Here's how the part is built. I have some questions about the finished solid (model axes, mm). A direction names the side the tool comes from. Coordinates: 2 decimals unless noted, no trailing zeros. Loops run counter-clockwise (first coordinate to the right, second up) from the corner with the lowest first, then second, coordinate; pieces in that order, holes last. Notation, with made-up numbers: (59.5, 23.25) -> (68.5, 23.25) arc R20 ccw to (68.5, 62.25) -> close; hole circle Ø4 at (27.25, 40). An arc over 180 degrees is marked (long way). Answer as a JSON object with one key per item and string values. Group by question number.
Q1. I want a section at A-A on y = -34.75. Write out the boundary of the cut face in (x, z).
Q2. I want a section at D-D on y = -46.75. Write out the boundary of the cut face in (x, z), then the cut area to 3 significant figures.
Q3. I want a section at C-C on z = 30.5. Write out the boundary of the cut face in (x, y).
Q4. I want a section at B-B on x = -3.25. Write out the boundary of the cut face in (y, z).
Q5. On a 3-axis mill with a long thin cutter (end or side, diameter ignored), from which of +Z, -Z, +X, -X, +Y, -Y can I reach the whole of each face in a straight line? I mean faces 1 (the flat face through (0, -25.266, 33)), 2 (the flat face through (-4, -35, 36)). Say none if no direction works.
Q6. Thinking about a two-plate mould opening in Z: for faces 3 (the cylindrical face through (0.06, -42.84, 21.7)), 4 (the cylindrical face through (-0.056, -38.763, 29.299)), 5 (the flat face through (0, -45.266, 33)), which applies, released by +Z, released by -Z, zero draft, split by the parting line, or undercut?
Q7. I need wall thicknesses on line 1 (Y direction, x = -1.75, z = 32.25); line 2 (Y direction, x = 2.5, z = 27.5); line 3 (Y direction, x = 2.75, z = 33.5). Which ranges of each line are inside material? Lowest first, please.
Q8. I'm going to push flat-ended pins straight in: pin 1 (2 mm diameter, centred on y = -33, z = 30.5, fed in from +X); pin 2 (4 mm diameter, centred on x = -0.5, y = -46.5, fed in from -Z); pin 3 (2.5 mm diameter, centred on x = 0, z = 32, fed in from -Y). Where does each tip first touch, or does it pass through?
```python
from build123d import *

# Parameters (mm, degrees)
F0_R          = 3.5
F1_DEPTH      = 4
F1_DEPTH_BACK = 4


with BuildPart() as f1:
    # F0 (on Right) → F1 (new body, two sides)
    with BuildSketch(Plane.YZ) as f1_sk:
        with BuildLine():
            Line((-20.266165, 46.737653), (-50.266165, 46.737653))
            Line((-50.266165, 46.737653), (-46.05444, 40.154854))
            ThreePointArc((-46.05444, 40.154854), (-45.467278, 38.863972), (-45.266165, 37.460161))
            Line((-45.266165, 37.460161), (-45.266165, 27.645153))
            ThreePointArc((-45.266165, 27.645153), (-42.776573, 21.634746), (-36.766165, 19.145153))
            Line((-36.766165, 19.145153), (-33.766165, 19.145153))
            ThreePointArc((-33.766165, 19.145153), (-27.755757, 21.634746), (-25.266165, 27.645153))
            Line((-25.266165, 27.645153), (-25.266165, 37.646666))
            ThreePointArc((-25.266165, 37.646666), (-25.055695, 39.082076), (-24.442004, 40.396642))
            Line((-24.442004, 40.396642), (-20.266165, 46.737653))
        make_face()
        with Locations((-35.266165, 29.145153)):
            Circle(F0_R, mode=Mode.SUBTRACT)
    extrude(amount=F1_DEPTH)
    extrude(f1_sk.sketch, amount=-F1_DEPTH_BACK)


solid = f1.part
```
Result set:
{
 "1": {"outline": "(-4, 19.15) -> (4, 19.15) -> (4, 25.68) -> (-4, 25.68) -> close; (-4, 32.61) -> (4, 32.61) -> (4, 46.74) -> (-4, 46.74) -> close"},
 "2": {"outline": "(-4, 41.24) -> (4, 41.24) -> (4, 46.74) -> (-4, 46.74) -> close", "area": "44.0 mm²"},
 "3": {"outline": "(-4, -45.27) -> (4, -45.27) -> (4, -38.49) -> (-4, -38.49) -> close; (-4, -32.04) -> (4, -32.04) -> (4, -25.27) -> (-4, -25.27) -> close"},
 "4": {"outline": "(-50.27, 46.74) -> (-46.05, 40.15) arc R5 cw to (-45.27, 37.46) -> (-45.27, 27.65) arc R8.5 ccw to (-36.77, 19.15) -> (-33.77, 19.15) arc R8.5 ccw to (-25.27, 27.65) -> (-25.27, 37.65) arc R5 cw to (-24.44, 40.4) -> (-20.27, 46.74) -> close; hole circle Ø7 at (-35.27, 29.15)"},
 "5": {"face 1": "-Z, +X, -X, +Y", "face 2": "+Z, -Z, -X, +Y, -Y"},
 "6": {"face 3": "released by -Z", "face 4": "undercut", "face 5": "zero draft"},
 "7": {"line 1": "y = -45.27 to -36.88, -33.65 to -25.27", "line 2": "y = -45.26 to -38.36, -32.18 to -25.27", "line 3": "y = -45.27 to -25.27"},
 "8": {"pin 1": "stops at x = 4", "pin 2": "stops at z = 24.12", "pin 3": "stops at y = -45.27"}
}
